```python
from build123d import *

# Parameters (mm, degrees)
F0_W     = 20
F0_H     = 40
F0_W_2   = 10
F0_H_2   = 30
F1_DEPTH = 40
F2_DEPTH = 5
F4_DEPTH = 60


with BuildPart() as f1:
    # F0 (on Top) → F1 (new body)
    with BuildSketch(Plane.XY):
        Rectangle(F0_W, F0_H)
        Rectangle(F0_W_2, F0_H_2, mode=Mode.SUBTRACT)
    extrude(amount=F1_DEPTH)

    # F0 (on Top) → F2 (join)
    with BuildSketch(Plane.XY):
        Rectangle(F0_W_2, F0_H_2)
    extrude(amount=F2_DEPTH)

    # F3 (on face) → F4 (cut)
    with BuildSketch(Plane.YZ.offset(10)):
        Polygon((-10, 10), (0, 10), (10, 10), (10, 30), (-10, 30), align=None)
    extrude(amount=-F4_DEPTH, mode=Mode.SUBTRACT)


solid = f1.part
```
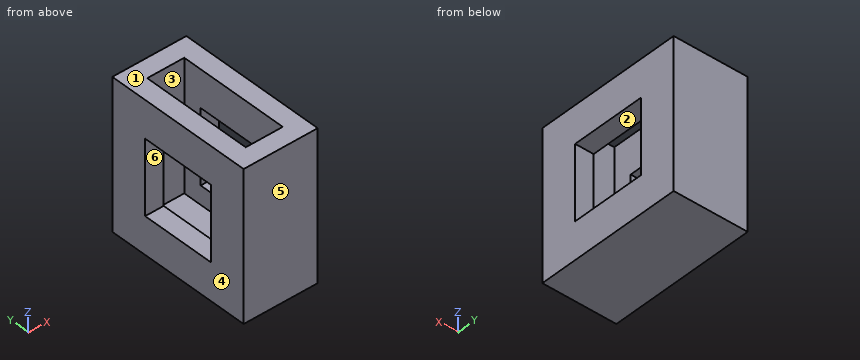
Verification items for the finished model (mm, model axes). Face numbers are marked on the shaded views. A direction names the side the tool comes from. Coordinates: 2 decimals unless noted, no trailing zeros. Order: outer loops, then holes, each group sorted by start corner. A loop starts at its lowest first (then second) coordinate and runs counter-clockwise, first axis right, second up. Notation, with made-up numbers: (-17.75, -37.5) -> (19.25, -37.5) arc R26 ccw to (19.25, 1.5) -> close; hole circle Ø4 at (-17.5, 40.25). An arc over 180 degrees is marked (long way). Put each result on its own line as item: value. Start each with the question number.
1) Cross-section at D-D (z = 36.5). Enter the section's corners in (x, y).
2) Cross-section at A-A (z = 18). Enter the section's corners in (x, y).
3) Tool access check on the marked faces 1, 2 and 3. Record the directions out of +Z, -Z, +X, -X, +Y, -Y that give a thin tool (end or side, any length) a straight path to the whole face; none if there is none.
4) Release check for a two-part mould opening along Y. For the marked faces 4, 5 and 6 record: pulls with the +Y half, pulls with the -Y half, needs draft (parallel to the pull), parting line crosses it, or undercut.
5) Go/stop test with a flat-tipped pin: pin 1 (3 mm diameter, centred on x = 0, y = 4.5, fed in from +Z). Record where the tip stops, or that it passes through.
6) Cross-section at C-C (x = 3.5). Enter the section's corners in (y, z).
7) Material ranges on L1, parallel to Y at x = -2, z = 13; L2, parallel to Z at x = 8, y = 2; L3, parallel to X at y = -2.5, z = 38.5, recorded low to high.
8) Cross-section at B-B (y = 4.5). Enter the section's corners in (x, z).
Geometry check:
1. outline: (-10, -20) -> (10, -20) -> (10, 20) -> (-10, 20) -> close; hole (-5, -15) -> (5, -15) -> (5, 15) -> (-5, 15) -> close
2. outline: (-10, -20) -> (10, -20) -> (10, -10) -> (5, -10) -> (5, -15) -> (-5, -15) -> (-5, -10) -> (-10, -10) -> close; (-10, 10) -> (-5, 10) -> (-5, 15) -> (5, 15) -> (5, 10) -> (10, 10) -> (10, 20) -> (-10, 20) -> close
3. face 1: +Z, +X, -X, +Y, -Y
3. face 2: +X, -X
3. face 3: +Z
4. face 4: needs draft
4. face 5: pulls with the -Y half
4. face 6: undercut
5. pin 1: stops at z = 5
6. outline: (-20, 0) -> (20, 0) -> (20, 40) -> (15, 40) -> (15, 5) -> (-15, 5) -> (-15, 40) -> (-20, 40) -> close
7. L1: y = -20 to -15, 15 to 20
7. L2: z = 0 to 10, 30 to 40
7. L3: x = -10 to -5, 5 to 10
8. outline: (-10, 0) -> (10, 0) -> (10, 10) -> (5, 10) -> (5, 5) -> (-5, 5) -> (-5, 10) -> (-10, 10) -> close; (-10, 30) -> (-5, 30) -> (-5, 40) -> (-10, 40) -> close; (5, 30) -> (10, 30) -> (10, 40) -> (5, 40) -> close
